```python
from build123d import *

# Parameters (mm, degrees)
BOSS_EXTRUDE1_DEPTH = 1219.2
FILLET1_R           = 0.4064
SKETCH4_W           = 1905.2
SKETCH4_H           = 103.278519729
CUT_EXTRUDE1_DEPTH  = 60
SKETCH5_W           = 2.47699065
SKETCH5_H           = 2.94685794
CUT_EXTRUDE2_DEPTH  = 600


with BuildPart() as part:
    # Sketch3 → Boss-Extrude1 (new, symmetric)
    with BuildSketch(Plane.XY):
        Polygon((3.175, 25.4), (0, 25.4), (0, 0), (25.4, 0), (25.4, 3.175), (3.175, 3.175), align=None)
    extrude(amount=BOSS_EXTRUDE1_DEPTH, both=True)

    # Fillet1
    fillet1_edges = [part.edges().sort_by_distance(p)[0] for p in [
        (3.175, 3.175, 0),
    ]]
    fillet(fillet1_edges, radius=FILLET1_R)

    # Sketch4 → Cut-Extrude1 (cut)
    with BuildSketch(Plane.ZY):
        with Locations((-266.6, -26.239259864)):
            Rectangle(SKETCH4_W, SKETCH4_H)
    extrude(amount=-CUT_EXTRUDE1_DEPTH, mode=Mode.SUBTRACT)

    # Sketch5 → Cut-Extrude2 (cut)
    with BuildSketch(Plane(origin=(0, 0, 686), x_dir=(-1, 0, 0), z_dir=(0, 0, -1))):
        with Locations((-4.413495325, 4.64842897)):
            Rectangle(SKETCH5_W, SKETCH5_H)
    extrude(amount=-CUT_EXTRUDE2_DEPTH, mode=Mode.SUBTRACT)


solid = part.part
```
Work out the finished part from the listing and answer in its coordinate system (mm). A direction names the side the tool comes from. Coordinates: 2 decimals unless noted, no trailing zeros. Write each loop counter-clockwise with the first axis right and the second up, starting at its lowest first coordinate (ties: lowest second). Pieces come first, ordered by that corner, then holes. Notation, with made-up numbers: (-2, 75.5) - (7, 75.5) arc R28 cw to (7, 110.5) - close; hole circle Ø8 at (-29.5, 29.25). An arc over 180 degrees is marked (long way). Answer as a JSON object with one key per item and string values.
Q1. Which of the six approach directions +Z, -Z, +X, -X, +Y, -Y give full straight-line access (tool end or side, diameter ignored) to faces 1 (the flat face through (0, 13, 956)), 2 (the flat face through (3.175, 14, 956))?
Results list:
{"face 1": "+Z, -Z, -X, +Y, -Y", "face 2": "+Z, -Z, +X, +Y"}
Q2. Given pin 1 Ø2 at (y, z) = (18.5, 1113.5) entering from -X; pin 2 Ø2 at (y, z) = (13, 832.5) entering from +X (3 decimals), each flat-ended and moving along its own axis, determine where each tip first touches the part or whether it passes through.
Results list:
{"pin 1": "stops at x = 0", "pin 2": "stops at x = 3.175"}
Q3. Consider L1, parallel to Y at x = 11.25, z = 920 (3 decimals). Determine where the line is inside the solid, lowest interval first. Write a range as from..to.
Results list:
{"L1": "y = 0..3.175"}
Q4. Find section B-B (z = 763). Write down the section's boundary in (x, y) (3 decimals).
Results list:
{"outline": "(0, 0) - (25.4, 0) - (25.4, 3.175) - (3.175, 3.175) - (3.175, 25.4) - (0, 25.4) - close"}
Q5. Find section A-A (x = 8.75). Write down the section's boundary in (y, z) (3 decimals), plus the area to 3 significant figures.
Results list:
{"outline": "(0, 686) - (3.175, 686) - (3.175, 1219.2) - (0, 1219.2) - close", "area": "1,690 mm^2"}
